```python
from build123d import *

# Parameters (mm, degrees)
F0_W     = 90
F0_H     = 120
F1_DEPTH = 5
F3_DEPTH = 5
F4_R     = 30
F4_R_2   = 3
F5_DEPTH = 5
F6_DEPTH = 5
F7_DEPTH = 10


with BuildPart() as f1:
    # F0 (on Front) → F1 (new body)
    with BuildSketch(Plane.XZ):
        with Locations((45, -60)):
            Rectangle(F0_W, F0_H)
    extrude(amount=F1_DEPTH)

    # F2 (on face) → F3 (join)
    with BuildSketch(Plane(origin=(0, 0, 0), x_dir=(-1, 0, 0), z_dir=(0, 1, 0))):
        with BuildLine():
            Line((-85, -104.8660687473), (-63, -114.8660687473))
            Line((-63, -114.8660687473), (-27, -114.8660687473))
            Line((-27, -114.8660687473), (-27, -109.8660687473))
            ThreePointArc((-27, -109.8660687473), (-21.8742088291, -98.5744789567), (-10, -95))
            Line((-10, -95), (-5, -95))
            Line((-5, -95), (-5, -24.8660687473))
            Line((-5, -24.8660687473), (-10, -24.8660687473))
            ThreePointArc((-10, -24.8660687473), (-21.8742088291, -21.2915897906), (-27, -10))
            Line((-27, -10), (-27, -5))
            Line((-27, -5), (-70, -5))
            ThreePointArc((-70, -5), (-80.6066017178, -9.3933982822), (-85, -20))
            Line((-85, -20), (-85, -104.8660687473))
        make_face()
    extrude(amount=F3_DEPTH)

    # F4 (on face) → F5 (cut)
    with BuildSketch(Plane(origin=(0, 5, 0), x_dir=(-1, 0, 0), z_dir=(0, 1, 0))):
        with Locations((-45, -60)):
            Circle(F4_R)
        with Locations((-59.14, -74.144270925)):
            Circle(F4_R_2, mode=Mode.SUBTRACT)
        with Locations((-65, -60)):
            Circle(F4_R_2, mode=Mode.SUBTRACT)
        with Locations((-45, -80)):
            Circle(F4_R_2, mode=Mode.SUBTRACT)
        with Locations((-30.86, -74.144270925)):
            Circle(F4_R_2, mode=Mode.SUBTRACT)
        with Locations((-25, -60)):
            Circle(F4_R_2, mode=Mode.SUBTRACT)
        with Locations((-59.14, -45.855729075)):
            Circle(F4_R_2, mode=Mode.SUBTRACT)
        with Locations((-45, -40)):
            Circle(F4_R_2, mode=Mode.SUBTRACT)
        with Locations((-30.86, -45.855729075)):
            Circle(F4_R_2, mode=Mode.SUBTRACT)
    extrude(amount=-F5_DEPTH, mode=Mode.SUBTRACT)

    # F6 (cut): a face of the model
    f6_faces = [f1.faces().sort_by_distance(p)[0] for p in [
        (25, 5, -60),
    ]]
    extrude(f6_faces, amount=-F6_DEPTH, mode=Mode.SUBTRACT)

    # F4 (on face) → F7 (cut)
    with BuildSketch(Plane(origin=(0, 5, 0), x_dir=(-1, 0, 0), z_dir=(0, 1, 0))):
        with Locations((-45, -80)):
            Circle(F4_R_2)
        with Locations((-30.86, -74.144270925)):
            Circle(F4_R_2)
        with Locations((-59.14, -45.855729075)):
            Circle(F4_R_2)
        with Locations((-65, -60)):
            Circle(F4_R_2)
        with Locations((-59.14, -74.144270925)):
            Circle(F4_R_2)
        with Locations((-30.86, -45.855729075)):
            Circle(F4_R_2)
        with Locations((-45, -40)):
            Circle(F4_R_2)
        with Locations((-25, -60)):
            Circle(F4_R_2)
    extrude(amount=-F7_DEPTH, mode=Mode.SUBTRACT)


solid = f1.part
```
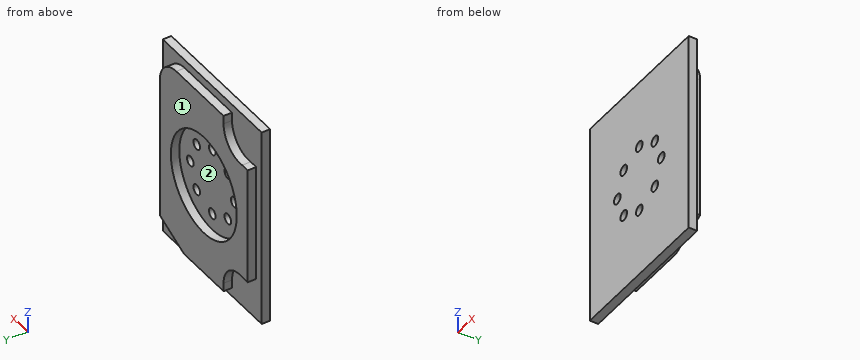
Here's how the part is built. I have some questions about the finished solid (model axes, mm). Face numbers are marked on the shaded views. Coordinates: 2 decimals unless noted, no trailing zeros. Write each loop counter-clockwise with the first axis right and the second up, starting at its lowest first coordinate (ties: lowest second). Pieces come first, ordered by that corner, then holes. Notation, with made-up numbers: M -32.5,67.5 L 15.5,67.5 A21 cw 15.5,71.5 Z; hole C 0,47.25 d10. An arc over 180 degrees is marked long. Answer as CSV lines item,"result". Start each with the question number.
Q1. Suppose I cut it at D-D, the plane x = 24. List the corners of the cut face in (y, z) for me, then the cut area to 3 significant figures.
Q2. Will these pins go through, and if not, where does the flat tip stop? pin 1 Ø5 at (x, z) = (45, -80) entering from +Y; pin 2 Ø5.5 at (y, z) = (3.5, -76.5) entering from +X; pin 3 Ø3 at (x, z) = (42.5, -84.5) entering from +Y; pin 4 Ø4 at (y, z) = (3.5, -44) entering from -X.
Q3. Suppose I cut it at B-B, the plane y = 3.25. List the corners of the cut face in (x, z) for me, then the cut area to 3 significant figures.
Q4. If we mould it in two halves opening along X, with no side actions, what happens to the marked faces 1 and 2? For each: pulls with the +X half, pulls with the -X half, needs draft (parallel to the pull), parting line crosses it, or undercut.
Q5. Suppose I cut it at C-C, the plane z = -75.5. List the corners of the cut face in (x, y) for me, then the cut area to 3 significant figures.
Q6. Suppose I cut it at A-A, the plane x = 45. List the corners of the cut face in (y, z) for me.
Q7. I need wall thicknesses on probe 1 along Z at (x, y) = (30.5, -4); probe 2 along Z at (x, y) = (59.14, -2.6); probe 3 along X at (y, z) = (-2.25, -71.5). Which ranges of each line are inside material? Lowest first, please. Write a range as [from, to].
Entries:
1,outline,"M -5,-120 L 0,-120 L 0,-100.87 L 5,-100.87 L 5,-81.42 L 0,-81.42 L 0,-62.83 L -5,-62.83 Z; M -5,-57.17 L 0,-57.17 L 0,-38.58 L 5,-38.58 L 5,-19 L 0,-19 L 0,0 L -5,0 Z"
1,area,"767 mm²"
2,pin 1,"passes through"
2,pin 2,"stops at x = 85"
2,pin 3,"stops at y = 0"
2,pin 4,"stops at x = 5"
3,outline,"M 5,-95 L 10,-95 A15 cw 27,-109.87 L 27,-114.87 L 63,-114.87 L 85,-104.87 L 85,-20 A15 ccw 70,-5 L 27,-5 L 27,-10 A15 cw 10,-24.87 L 5,-24.87 Z; hole C 45,-60 d60"
3,area,"5,020 mm²"
4,face 1,"needs draft"
4,face 2,"undercut"
5,outline,"M 0,-5 L 28.18,-5 L 28.18,0 L 19.31,0 L 19.31,5 L 5,5 L 5,0 L 0,0 Z; M 33.54,-5 L 56.46,-5 L 56.46,0 L 33.54,0 Z; M 61.82,-5 L 90,-5 L 90,0 L 85,0 L 85,5 L 70.69,5 L 70.69,0 L 61.82,0 Z"
5,area,"540 mm²"
6,outline,"M -5,-120 L 0,-120 L 0,-114.87 L 5,-114.87 L 5,-90 L 0,-90 L 0,-83 L -5,-83 Z; M -5,-77 L 0,-77 L 0,-43 L -5,-43 Z; M -5,-37 L 0,-37 L 0,-30 L 5,-30 L 5,-5 L 0,-5 L 0,0 L -5,0 Z"
7,probe 1,"z = [-120, -77.12], [-71.17, -48.83], [-42.88, 0]"
7,probe 2,"z = [-120, -77.14], [-71.14, -48.86], [-42.86, 0]"
7,probe 3,"x = [0, 29.44], [32.28, 57.72], [60.56, 90]"
